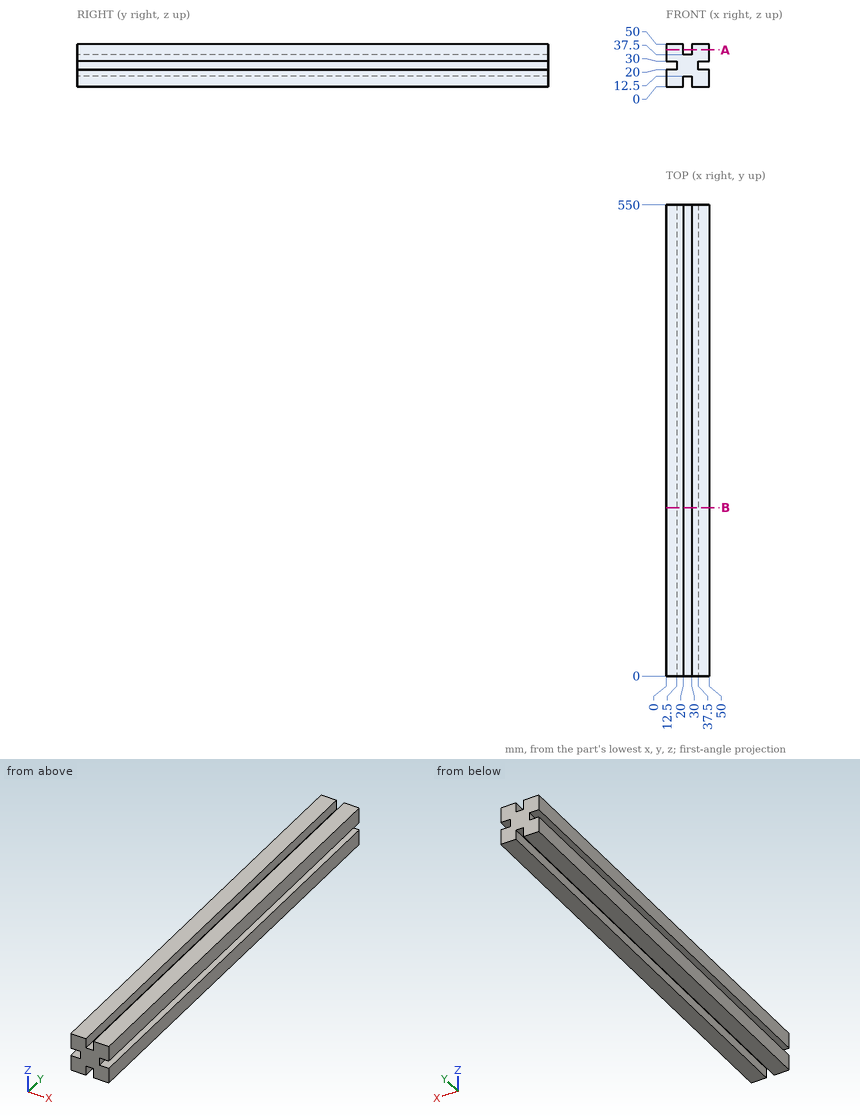
Study the drawing (mm; zero at the part's minimum x, y, z) and answer. Give positions to 0.01 mm unless a question says otherwise; leave off trailing zeros. Loops run counter-clockwise (first coordinate to the right, second up) from the corner with the lowest first, then second, coordinate; pieces in that order, holes last. Notation, with made-up numbers: (49, 29) - (107, 29) arc R30 cw to (107, 52) - close; hole circle Ø8 at (58.25, 6). An arc over 180 degrees is marked (long way). One line per question, with ' | ' between items.
(1) Straight lines are drawn through the part: probe 1 along Z at (x, y) = (11, 250.5); probe 2 along X at (y, z) = (231, 29.5). For each, find the intervals that lie inside material, in ascending order.
Recorded:
probe 1: z = 0 to 20, 30 to 50 | probe 2: x = 12.5 to 37.5
(2) Each of these flat-tipped pins is pushed along its axis until it touches: pin 1 Ø10 at (y, z) = (295.5, 39.5) entering from -X; pin 2 Ø1 at (y, z) = (142.5, 23) entering from -X; pin 3 Ø8 at (y, z) = (215.5, 24.5) entering from +X. Where does it stop, or does it pass through?
Recorded:
pin 1: stops at x = 0 | pin 2: stops at x = 12.5 | pin 3: stops at x = 37.5
(3) The part is cut by section B-B (y = 196.5). Write down the section's boundary in (x, z), then the cut area to 3 significant figures.
Recorded:
outline: (0, 0) - (20, 0) - (20, 12.5) - (30, 12.5) - (30, 0) - (50, 0) - (50, 20) - (37.5, 20) - (37.5, 30) - (50, 30) - (50, 50) - (30, 50) - (30, 37.5) - (20, 37.5) - (20, 50) - (0, 50) - (0, 30) - (12.5, 30) - (12.5, 20) - (0, 20) - close | area: 2,000 mm²
(4) The part is cut by section A-A (z = 43). Write down the section's boundary in (x, y), then the cut area to 3 significant figures.
Recorded:
outline: (0, 0) - (20, 0) - (20, 550) - (0, 550) - close; (30, 0) - (50, 0) - (50, 550) - (30, 550) - close | area: 22,000 mm²
